```python
from build123d import *

# Parameters (mm, degrees)
SKETCH1_R           = 1.4
BOSS_EXTRUDE1_DEPTH = 1.6
SKETCH2_W           = 20
SKETCH2_H           = 15.9
BOSS_EXTRUDE2_DEPTH = 13.5
SKETCH3_W           = 16
SKETCH3_H           = 13.1
BOSS_EXTRUDE3_DEPTH = 14.8
SKETCH4_W           = 6
SKETCH4_H           = 16.9
BOSS_EXTRUDE4_DEPTH = 6
SKETCH6_W           = 19.946979578
SKETCH6_H           = 15.036953836
BOSS_EXTRUDE5_DEPTH = 1


with BuildPart() as part:
    # Sketch1 → Boss-Extrude1 (new body)
    with BuildSketch(Plane(origin=(0, 0, 0), x_dir=(1, 0, 0), z_dir=(0, 1, 0))):
        with BuildLine():
            Line((-39, 28), (39, 28))
            ThreePointArc((39, 28), (41.474873734, 26.974873734), (42.5, 24.5))
            Line((42.5, 24.5), (42.5, -24.5))
            ThreePointArc((42.5, -24.5), (41.474873734, -26.974873734), (39, -28))
            Line((39, -28), (-39, -28))
            ThreePointArc((-39, -28), (-41.474873734, -26.974873734), (-42.5, -24.5))
            Line((-42.5, -24.5), (-42.5, 24.5))
            ThreePointArc((-42.5, 24.5), (-41.474873734, 26.974873734), (-39, 28))
        make_face()
        with Locations(Location((-39, 24.5, 0), (0, 0, 270))):
            Circle(SKETCH1_R, mode=Mode.SUBTRACT)
        with Locations(Location((19, 24.5, 0), (0, 0, 270))):
            Circle(SKETCH1_R, mode=Mode.SUBTRACT)
        with Locations(Location((19, -24.5, 0), (0, 0, 90))):
            Circle(SKETCH1_R, mode=Mode.SUBTRACT)
        with Locations(Location((-39, -24.5, 0), (0, 0, 90))):
            Circle(SKETCH1_R, mode=Mode.SUBTRACT)
    extrude(amount=BOSS_EXTRUDE1_DEPTH)

    # Sketch2 → Boss-Extrude2 (add)
    with BuildSketch(Plane(origin=(0, 1.6, 0), x_dir=(1, 0, 0), z_dir=(0, 1, 0))):
        with Locations((34.6, -17.75)):
            Rectangle(SKETCH2_W, SKETCH2_H)
    extrude(amount=BOSS_EXTRUDE2_DEPTH)

    # Sketch3 → Boss-Extrude3 (add)
    with BuildSketch(Plane(origin=(0, 1.6, 0), x_dir=(1, 0, 0), z_dir=(0, 1, 0))):
        with Locations((36.6, 0.95)):
            Rectangle(SKETCH3_W, SKETCH3_H)
        with Locations((36.6, 18.95)):
            Rectangle(SKETCH3_W, SKETCH3_H)
    extrude(amount=BOSS_EXTRUDE3_DEPTH)

    # Sketch4 → Boss-Extrude4 (add)
    with BuildSketch(Plane(origin=(0, 1.6, 0), x_dir=(1, 0, 0), z_dir=(0, 1, 0))):
        with Locations((11, -19.55)):
            Rectangle(SKETCH4_W, SKETCH4_H)
    extrude(amount=BOSS_EXTRUDE4_DEPTH)

    # Sketch6 → Boss-Extrude5 (add)
    with BuildSketch(Plane(origin=(0, 1.6, 0), x_dir=(1, 0, 0), z_dir=(0, 1, 0))):
        with Locations((-12.912885705, 1.636675247)):
            Rectangle(SKETCH6_W, SKETCH6_H)
    extrude(amount=BOSS_EXTRUDE5_DEPTH)


solid = part.part
```
Here's how the part is built. I have some questions about the finished solid (model axes, mm). A direction names the side the tool comes from. Round coordinates to 2 decimals unless told otherwise and drop trailing zeros. Order: outer loops, then holes, each group sorted by start corner. A loop starts at its lowest first (then second) coordinate and runs counter-clockwise, first axis right, second up. Notation, with made-up numbers: M 22.5,-27 L 76.5,-27 A9 cw 76.5,-22 Z; hole C 81,41 d1. An arc over 180 degrees is marked long. Answer as CSV lines item,"result".
Item 1: Please list where these lines run through material, in increasing order: L1, parallel to X at y = 0.75, z = 24.5; L2, parallel to Z at x = 29.5, y = 2.25; L3, parallel to X at y = 2, z = 1.5. Write a range as [from, to].
From the geometry:
L1,"[-42.5, -40.4], [-37.6, 17.6], [20.4, 42.5]"
L2,"[-25.5, -12.4], [-7.5, 5.6], [9.8, 25.7]"
L3,"[-22.89, -2.94], [28.6, 44.6]"
Item 2: Imagine slicing it at A-A on x = 19. List the corners of the cut face in (y, z) for me, and give its area (3 significant figures).
From the geometry:
outline,"M 0,-28 L 1.6,-28 L 1.6,-25.9 L 0,-25.9 Z; M 0,-23.1 L 1.6,-23.1 L 1.6,23.1 L 0,23.1 Z; M 0,25.9 L 1.6,25.9 L 1.6,28 L 0,28 Z"
area,"80.6 mm2"
Item 3: Imagine slicing it at B-B on y = 4.25. List the corners of the cut face in (x, z) for me, and give its area (3 significant figures).
From the geometry:
outline,"M 8,11.1 L 14,11.1 L 14,28 L 8,28 Z; M 24.6,9.8 L 44.6,9.8 L 44.6,25.7 L 24.6,25.7 Z; M 28.6,-25.5 L 44.6,-25.5 L 44.6,-12.4 L 28.6,-12.4 Z; M 28.6,-7.5 L 44.6,-7.5 L 44.6,5.6 L 28.6,5.6 Z"
area,"839 mm2"
Item 4: Imagine slicing it at D-D on x = 33.5. List the corners of the cut face in (y, z) for me, and give its area (3 significant figures).
From the geometry:
outline,"M 0,-28 L 1.6,-28 L 1.6,-25.5 L 16.4,-25.5 L 16.4,-12.4 L 1.6,-12.4 L 1.6,-7.5 L 16.4,-7.5 L 16.4,5.6 L 1.6,5.6 L 1.6,9.8 L 15.1,9.8 L 15.1,25.7 L 1.6,25.7 L 1.6,28 L 0,28 Z"
area,"692 mm2"
Item 5: For pin 1 (6 mm diameter, centred on y = 7.5, z = -18.5, fed in from -X); pin 2 (1.8 mm diameter, centred on x = 44, z = 15, fed in from -Y); pin 3 (1.3 mm diameter, centred on y = 0.5, z = 6, fed in from +X); pin 4 (4 mm diameter, centred on x = -31, y = 4, fed in from +Z), each with a flat end and sliding along its axis, tell me the tip position at first contact or that it passes through.
From the geometry:
pin 1,"x = 28.6"
pin 2,"y = 1.6"
pin 3,"x = 42.5"
pin 4,"through"
Item 6: We'd pull the mould along Z, two halves only. Please class faces 1 (the flat face through (36, 9, -25.5)), 2 (the flat face through (34, 8, 9.8)), 3 (the flat face through (44.6, 9, -19)): +Z half, -Z half, draft (parallel to the pull), parting line (faces both ways), or undercut.
From the geometry:
face 1,"-Z half"
face 2,"undercut"
face 3,"draft"
Item 7: Which directions (+Z, -Z, +X, -X, +Y, -Y) give clear straight access to the entire face, cutting with the end or side of a thin tool? Please do faces 4 (the flat face through (11, 7.6, 19)), 5 (the flat face through (11, 5, 11.1)), 6 (the cylindrical face through (41.5, 0.79, 26.95)), 7 (the flat face through (34, 8, 25.7)).
From the geometry:
face 4,"+Z, -Z, -X, +Y"
face 5,"-Z, -X, +Y"
face 6,"+Z, +X, -Y"
face 7,"+Z, +X, +Y"
Item 8: Imagine slicing it at C-C on y = 12.25. List the corners of the cut face in (x, z) for me, and give its area (3 significant figures).
From the geometry:
outline,"M 24.6,9.8 L 44.6,9.8 L 44.6,25.7 L 24.6,25.7 Z; M 28.6,-25.5 L 44.6,-25.5 L 44.6,-12.4 L 28.6,-12.4 Z; M 28.6,-7.5 L 44.6,-7.5 L 44.6,5.6 L 28.6,5.6 Z"
area,"737 mm2"
